from build123d import *

# Parameters (mm, degrees)
F1_DEPTH       = 30
F2_W           = 35
F2_H           = 50
F3_DEPTH       = 15.001
F5_D           = 5.5
F5_CSINK_D     = 11.2
F5_CSINK_ANGLE = 90
F4_R           = 10
F6_DEPTH       = 5
F7_R           = 8.3224131339
F8_DEPTH       = 5


with BuildPart() as f1:
    # F0 (on Front) → F1 (new body, symmetric)
    with BuildSketch(Plane.XZ):
        Polygon((50, 45), (50, 60), (0, 60), (0, 0), (60, 0), (60, 15), (15, 15), (15, 45), align=None)
    extrude(amount=F1_DEPTH, both=True)

    # F2 (on face) → F3 (cut, through all)
    with BuildSketch(Plane.XY.offset(15)):
        with Locations((37.5, 0)):
            Rectangle(F2_W, F2_H)
    extrude(amount=-F3_DEPTH, mode=Mode.SUBTRACT)

    # F5 (through all)
    with Locations(Plane.XY.offset(60)):
        with Locations((25, -14)):
            CounterSinkHole(F5_D / 2, F5_CSINK_D / 2, counter_sink_angle=F5_CSINK_ANGLE)

    # F4 (on face) → F6 (join)
    with BuildSketch(Plane.XY.offset(60)):
        with Locations((25, 14)):
            Circle(F4_R)
    extrude(amount=F6_DEPTH)

    # F7 (on face) → F8 (join)
    with BuildSketch(Plane.XY.offset(65)):
        with Locations((25, 14)):
            Circle(F7_R)
    extrude(amount=-F8_DEPTH)


solid = f1.part
Geometry check sheet. Reference: the model listing, model coordinates, mm. A direction names the side the tool comes from. Give positions to 0.01 mm unless a question says otherwise; leave off trailing zeros. Loops run counter-clockwise (first coordinate to the right, second up) from the corner with the lowest first, then second, coordinate; pieces in that order, holes last. Notation, with made-up numbers: (-2, 30.25) -> (8, 30.25) arc R20 ccw to (8, 50.25) -> close; hole circle Ø1 at (32, -17). An arc over 180 degrees is marked (long way). Answer in a Markdown table with one row per item. Add a question column.
1) Material ranges on probe 1 along Y at (x, z) = (25, 50); probe 2 along X at (y, z) = (7, 14); probe 3 along Y at (x, z) = (27, 10), recorded low to high. Write a range as from..to.
2) Cross-section at D-D on z = 13.5. Record the boundary of the cut face in (x, y), and give its area (3 significant figures).
3) Cross-section at B-B on x = 52. Record the boundary of the cut face in (y, z), and give its area (3 significant figures).
4) Set-up check for faces 1 (the face through (55, 0, 8)), 2 (the face through (50, 0, 52)), 3 (the face through (34.54, 17, 62.46)), 4 (the face through (20, 0, 8)), 5 (the face through (58, 0, 15)): record each of +Z, -Z, +X, -X, +Y, -Y from which the full face is reachable in a straight line by a thin tool's end or side.
5) Gauge pin test, flat ends, axial feed: P1, Ø5, axis at x = 25, y = -14, coming from the -Z side; P2, Ø7.5, axis at y = -11, z = 54.5, coming from the +X side; P3, Ø8, axis at x = 37, y = 22.5, coming from the +Z side; P4, Ø5, axis at x = 28, y = -15, coming from the -Z side. Record the tip position at first contact, or that the pin passes through.
6) Draft check along X on faces 6 (the face through (0, 0, 30)), 7 (the face through (25, 14, 65)), 8 (the face through (27.747, -13.879, 50.99)). Enter one of: pulls with the +X half, pulls with the -X half, needs draft (parallel to the pull), parting line crosses it, or undercut.
7) Cross-section at A-A on y = 20. Record the boundary of the cut face in (x, z).
8) Cross-section at C-C on y = -14. Record the boundary of the cut face in (x, z).
Outcome:
| question | item | result |
|---|---|---|
| 1 | probe 1 | y = -30..-16.75, -11.25..30 |
| 1 | probe 2 | x = 0..20, 55..60 |
| 1 | probe 3 | y = -30..-25, 25..30 |
| 2 | outline | (0, -30) -> (60, -30) -> (60, 30) -> (0, 30) -> close; hole (20, -25) -> (55, -25) -> (55, 25) -> (20, 25) -> close |
| 2 | area | 1,850 mm^2 |
| 3 | outline | (-30, 0) -> (-25, 0) -> (-25, 15) -> (-30, 15) -> close; (25, 0) -> (30, 0) -> (30, 15) -> (25, 15) -> close |
| 3 | area | 150 mm^2 |
| 4 | face 1 | +Z, -Z |
| 4 | face 2 | +Z, +X, +Y, -Y |
| 4 | face 3 | +Z |
| 4 | face 4 | -Z |
| 4 | face 5 | +X, +Y, -Y |
| 5 | P1 | passes through |
| 5 | P2 | stops at x = 50 |
| 5 | P3 | stops at z = 60 |
| 5 | P4 | stops at z = 45 |
| 6 | face 6 | pulls with the -X half |
| 6 | face 7 | needs draft |
| 6 | face 8 | undercut |
| 7 | outline | (0, 0) -> (20, 0) -> (20, 15) -> (15, 15) -> (15, 45) -> (50, 45) -> (50, 60) -> (33, 60) -> (33, 65) -> (17, 65) -> (17, 60) -> (0, 60) -> close; (55, 0) -> (60, 0) -> (60, 15) -> (55, 15) -> close |
| 8 | outline | (0, 0) -> (20, 0) -> (20, 15) -> (15, 15) -> (15, 45) -> (22.25, 45) -> (22.25, 57.15) -> (19.4, 60) -> (0, 60) -> close; (27.75, 45) -> (50, 45) -> (50, 60) -> (30.6, 60) -> (27.75, 57.15) -> close; (55, 0) -> (60, 0) -> (60, 15) -> (55, 15) -> close |
